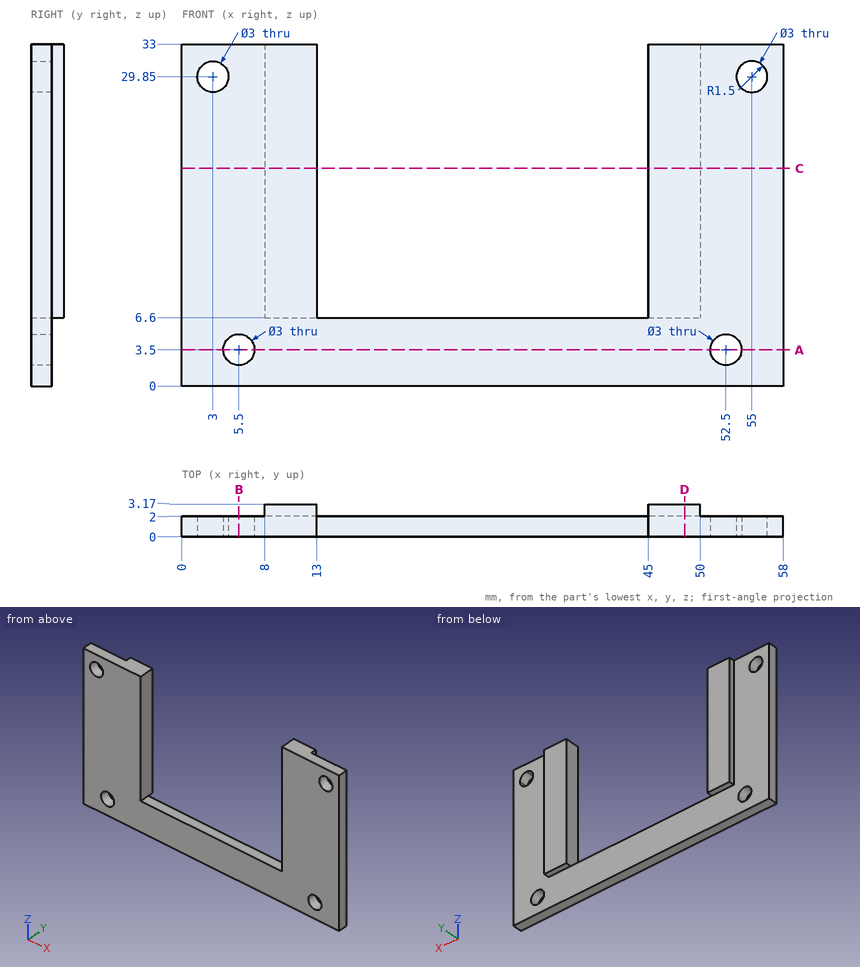
Part print with two shaded views. Sizes in mm from the minimum x, y, z corner. Coordinates: 2 decimals unless noted, no trailing zeros. Order: outer loops, then holes, each group sorted by start corner. A loop starts at its lowest first (then second) coordinate and runs counter-clockwise, first axis right, second up. Notation, with made-up numbers: (31.25, 46) - (84.25, 46) arc R17 ccw to (84.25, 61) - close; hole circle Ø7 at (-30, -23.5). An arc over 180 degrees is marked (long way). Answer in a Markdown table with one row per item.
1. Slice it at A-A, the plane z = 3.5. List the corners of the cut face in (x, y).
Answer:
| item | result |
|---|---|
| outline | (0, 0) - (4, 0) - (4, 2) - (0, 2) - close; (7, 0) - (51, 0) - (51, 2) - (7, 2) - close; (54, 0) - (58, 0) - (58, 2) - (54, 2) - close |
2. Slice it at B-B, the plane x = 5.5. List the corners of the cut face in (y, z).
Answer:
| item | result |
|---|---|
| outline | (0, 0) - (2, 0) - (2, 2) - (0, 2) - close; (0, 5) - (2, 5) - (2, 33) - (0, 33) - close |
3. Flat gauge pins, fed straight in: P1, Ø5, axis at x = 3, z = 29.85, coming from the +Y side; P2, Ø1.3, axis at x = 10.5, y = 3, coming from the -Z side; P3, Ø1, axis at x = 14.5, y = 2, coming from the +Z side. Where does each tip first touch, or does it go through?
Answer:
| item | result |
|---|---|
| P1 | y = 2 |
| P2 | z = 6.6 |
| P3 | z = 6.6 |
4. Slice it at C-C, the plane z = 21. List the corners of the cut face in (x, y), then the cut area to 3 significant figures.
Answer:
| item | result |
|---|---|
| outline | (0, 0) - (13, 0) - (13, 3.17) - (8, 3.17) - (8, 2) - (0, 2) - close; (45, 0) - (58, 0) - (58, 2) - (50, 2) - (50, 3.17) - (45, 3.17) - close |
| area | 63.7 mm² |
5. Drill centre lines: L1, parallel to X at y = 0.7, z = 29.85; L2, parallel to X at y = 0.65, z = 3.5; L3, parallel to X at y = 2.5, z = 23. Where is each one in solid material? Low to high. Write a range as from..to.
Answer:
| item | result |
|---|---|
| L1 | 0..1.5, 4.5..13, 45..53.5, 56.5..58 |
| L2 | 0..4, 7..51, 54..58 |
| L3 | 8..13, 45..50 |
6. Slice it at D-D, the plane x = 48.5. List the corners of the cut face in (y, z).
Answer:
| item | result |
|---|---|
| outline | (0, 0) - (2, 0) - (2, 6.6) - (3.17, 6.6) - (3.17, 33) - (0, 33) - close |
